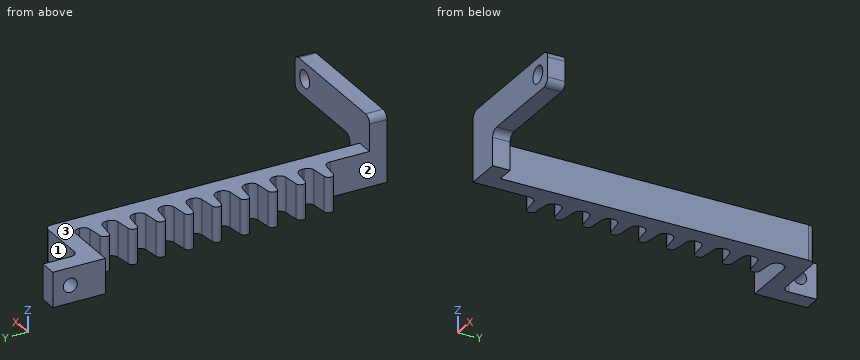
from build123d import *

# Parameters (mm, degrees)
BOSS_EXTRUDE1_DEPTH    = 7
SKETCH2_W              = 5
SKETCH2_H              = 10
BOSS_EXTRUDE2_DEPTH    = 95
SKETCH15_R             = 3.5
CUT_EXTRUDE3_DEPTH     = 7
SKETCH18_W             = 10
SKETCH18_H             = 5
BOSS_EXTRUDE3_DEPTH    = 34
BOSS_EXTRUDE4_DEPTH    = 10
FILLET1_R              = 2
FILLET2_R              = 2
LPATTERN2_COUNT        = 9
LPATTERN2_PITCH        = 8
FILLET1_OF_LPATTERN2_R = 2
SKETCH20_R             = 2.5
CUT_EXTRUDE4_DEPTH     = 10
CIRPATTERN2_COUNT      = 4
SKETCH22_W             = 135.679550384
SKETCH22_H             = 112.96527187
CUT_EXTRUDE5_DEPTH     = 61.740758688
BOSS_EXTRUDE5_START    = 5
SKETCH23_R             = 2.5
BOSS_EXTRUDE5_DEPTH    = 5
CUT_EXTRUDE6_START     = -10
CUT_EXTRUDE6_DEPTH     = 10
SKETCH27_W             = 10
SKETCH27_H             = 5
BOSS_EXTRUDE6_DEPTH    = 5
SKETCH28_W             = 5
SKETCH28_H             = 10
BOSS_EXTRUDE7_DEPTH    = 10
SKETCH29_R             = 2
CUT_EXTRUDE7_DEPTH     = 5
FILLET3_R              = 2


with BuildPart() as part:
    # Sketch1 → Boss-Extrude1 (new body)
    with BuildSketch(Plane(origin=(0, 0, 0), x_dir=(1, 0, 0), z_dir=(0, 1, 0))):
        with BuildLine():
            Line((-8, 56.940758688), (-8, 59.740758688))
            ThreePointArc((-8, 59.740758688), (-7.414213562, 61.154972251), (-6, 61.740758688))
            Line((-6, 61.740758688), (6, 61.740758688))
            ThreePointArc((6, 61.740758688), (7.414213562, 61.154972251), (8, 59.740758688))
            Line((8, 59.740758688), (8, 56.940758688))
            ThreePointArc((8, 56.940758688), (22.004297361, 53.123073119), (34.606342345, 45.920050844))
            Line((34.606342345, 45.920050844), (36.586241332, 47.899949831))
            ThreePointArc((36.586241332, 47.899949831), (38.000454895, 48.485736269), (39.414668457, 47.899949831))
            Line((39.414668457, 47.899949831), (47.899949831, 39.414668457))
            ThreePointArc((47.899949831, 39.414668457), (48.485736269, 38.000454895), (47.899949831, 36.586241332))
            Line((47.899949831, 36.586241332), (45.920050844, 34.606342345))
            ThreePointArc((45.920050844, 34.606342345), (53.123073119, 22.004297361), (56.940758688, 8))
            Line((56.940758688, 8), (59.740758688, 8))
            ThreePointArc((59.740758688, 8), (61.154972251, 7.414213562), (61.740758688, 6))
            Line((61.740758688, 6), (61.740758688, -6))
            ThreePointArc((61.740758688, -6), (61.154972251, -7.414213562), (59.740758688, -8))
            Line((59.740758688, -8), (56.940758688, -8))
            ThreePointArc((56.940758688, -8), (53.123073119, -22.004297361), (45.920050844, -34.606342345))
            Line((45.920050844, -34.606342345), (47.899949831, -36.586241332))
            ThreePointArc((47.899949831, -36.586241332), (48.485736269, -38.000454895), (47.899949831, -39.414668457))
            Line((47.899949831, -39.414668457), (39.414668457, -47.899949831))
            ThreePointArc((39.414668457, -47.899949831), (38.000454895, -48.485736269), (36.586241332, -47.899949831))
            Line((36.586241332, -47.899949831), (34.606342345, -45.920050844))
            ThreePointArc((34.606342345, -45.920050844), (22.004297361, -53.123073119), (8, -56.940758688))
            Line((8, -56.940758688), (8, -59.740758688))
            ThreePointArc((8, -59.740758688), (7.414213562, -61.154972251), (6, -61.740758688))
            Line((6, -61.740758688), (-6, -61.740758688))
            ThreePointArc((-6, -61.740758688), (-7.414213562, -61.154972251), (-8, -59.740758688))
            Line((-8, -59.740758688), (-8, -56.940758688))
            ThreePointArc((-8, -56.940758688), (-22.004297361, -53.123073119), (-34.606342345, -45.920050844))
            Line((-34.606342345, -45.920050844), (-36.586241332, -47.899949831))
            ThreePointArc((-36.586241332, -47.899949831), (-38.000454895, -48.485736269), (-39.414668457, -47.899949831))
            Line((-39.414668457, -47.899949831), (-47.899949831, -39.414668457))
            ThreePointArc((-47.899949831, -39.414668457), (-48.485736269, -38.000454895), (-47.899949831, -36.586241332))
            Line((-47.899949831, -36.586241332), (-45.920050844, -34.606342345))
            ThreePointArc((-45.920050844, -34.606342345), (-53.123073119, -22.004297361), (-56.940758688, -8))
            Line((-56.940758688, -8), (-59.740758688, -8))
            ThreePointArc((-59.740758688, -8), (-61.154972251, -7.414213562), (-61.740758688, -6))
            Line((-61.740758688, -6), (-61.740758688, 6))
            ThreePointArc((-61.740758688, 6), (-61.154972251, 7.414213562), (-59.740758688, 8))
            Line((-59.740758688, 8), (-56.940758688, 8))
            ThreePointArc((-56.940758688, 8), (-53.123073119, 22.004297361), (-45.920050844, 34.606342345))
            Line((-45.920050844, 34.606342345), (-47.899949831, 36.586241332))
            ThreePointArc((-47.899949831, 36.586241332), (-48.485736269, 38.000454895), (-47.899949831, 39.414668457))
            Line((-47.899949831, 39.414668457), (-39.414668457, 47.899949831))
            ThreePointArc((-39.414668457, 47.899949831), (-38.000454895, 48.485736269), (-36.586241332, 47.899949831))
            Line((-36.586241332, 47.899949831), (-34.606342345, 45.920050844))
            ThreePointArc((-34.606342345, 45.920050844), (-22.004297361, 53.123073119), (-8, 56.940758688))
        make_face()
    extrude(amount=BOSS_EXTRUDE1_DEPTH)

    # Sketch2 → Boss-Extrude2 (add)
    with BuildSketch(Plane(origin=(0, 7, 0), x_dir=(1, 0, 0), z_dir=(0, 1, 0))):
        with Locations((19.5, 10)):
            Rectangle(SKETCH2_W, SKETCH2_H)
        with Locations((-19.5, 10)):
            Rectangle(SKETCH2_W, SKETCH2_H)
    extrude(amount=BOSS_EXTRUDE2_DEPTH)

    # Sketch15 → Cut-Extrude3 (cut)
    with BuildSketch(Plane.XZ):
        with Locations(Location((0, 0, 0), (0, 0, 270))):
            Circle(SKETCH15_R)
    extrude(amount=-CUT_EXTRUDE3_DEPTH, mode=Mode.SUBTRACT)

    # Sketch18 → Boss-Extrude3 (add)
    with BuildSketch(Plane(origin=(-17, 0, 0), x_dir=(0, 0, -1), z_dir=(1, 0, 0))):
        with Locations((10, 99.5)):
            Rectangle(SKETCH18_W, SKETCH18_H)
    extrude(amount=BOSS_EXTRUDE3_DEPTH)

    # Sketch19 → Boss-Extrude4 (add)
    with BuildSketch(Plane(origin=(0, 0, -15), x_dir=(-1, 0, 0), z_dir=(0, 0, -1))):
        with BuildLine():
            Line((-17, 93), (-11.04472309, 92.26878394))
            ThreePointArc((-11.04472309, 92.26878394), (-9.922197884, 91), (-11.04472309, 89.73121606))
            Line((-11.04472309, 89.73121606), (-17, 89))
            Line((-17, 89), (-17, 93))
        make_face()
    boss_extrude4 = extrude(amount=-BOSS_EXTRUDE4_DEPTH)

    # Fillet1
    fillet1_edges = [part.edges().sort_by_distance(p)[0] for p in [
        (17, 89, -10),
        (17, 93, -10),
    ]]
    fillet(fillet1_edges, radius=FILLET1_R)

    # Fillet2
    fillet2_edges = [part.edges().sort_by_distance(p)[0] for p in [
        (22, 102, -10),
        (-22, 102, -10),
        (-17, 97, -10),
        (17, 97, -10),
    ]]
    fillet(fillet2_edges, radius=FILLET2_R)

    # LPattern2: Boss-Extrude4 ×9
    with Locations(*[(0, -i * LPATTERN2_PITCH, 0) for i in range(1, LPATTERN2_COUNT)]):
        add(boss_extrude4)

    # Fillet1 of LPattern2
    fillet1_of_lpattern2_edges = [part.edges().sort_by_distance(p)[0] for p in [
        (17, 81, -10),
        (17, 85, -10),
        (17, 73, -10),
        (17, 77, -10),
        (17, 65, -10),
        (17, 69, -10),
        (17, 57, -10),
        (17, 61, -10),
        (17, 49, -10),
        (17, 53, -10),
        (17, 41, -10),
        (17, 45, -10),
        (17, 33, -10),
        (17, 37, -10),
        (17, 25, -10),
        (17, 29, -10),
    ]]
    fillet(fillet1_of_lpattern2_edges, radius=FILLET1_OF_LPATTERN2_R)

    # Sketch20 → Cut-Extrude4 (cut)
    with BuildSketch(Plane(origin=(0, 7, 0), x_dir=(1, 0, 0), z_dir=(0, 1, 0))):
        with Locations(Location((0, 50, 0), (0, 0, 270))):
            Circle(SKETCH20_R)
    cut_extrude4 = extrude(amount=-CUT_EXTRUDE4_DEPTH, mode=Mode.SUBTRACT)

    # CirPattern2: Cut-Extrude4 ×4 about axis
    cirpattern2_axis = Axis((0, 0, 0), (0, 1, 0))
    for i in range(1, CIRPATTERN2_COUNT):
        add(cut_extrude4.rotate(cirpattern2_axis, i * 360 / CIRPATTERN2_COUNT), mode=Mode.SUBTRACT)

    # Sketch22 → Cut-Extrude5 (cut)
    with BuildSketch(Plane(origin=(0, 0, 0), x_dir=(0, 0, -1), z_dir=(1, 0, 0))):
        with Locations((-0.132373771, 50.371775874)):
            Rectangle(SKETCH22_W, SKETCH22_H)
    extrude(amount=-CUT_EXTRUDE5_DEPTH, mode=Mode.SUBTRACT)

    # Sketch23 → Boss-Extrude5 (add)
    with BuildSketch(Plane(origin=(0, 7, 0), x_dir=(1, 0, 0), z_dir=(0, 1, 0)).offset(BOSS_EXTRUDE5_START)):
        with BuildLine():
            Line((55, 3), (55, -2.687123684))
            ThreePointArc((55, -2.687123684), (54.414213562, -4.101337246), (53, -4.687123684))
            Line((53, -4.687123684), (19, -4.687123684))
            ThreePointArc((19, -4.687123684), (17.585786438, -4.101337246), (17, -2.687123684))
            Line((17, -2.687123684), (17, 5))
            Line((17, 5), (53, 5))
            ThreePointArc((53, 5), (54.414213562, 4.414213562), (55, 3))
        make_face()
        with Locations(Location((50, 0, 0), (0, 0, 270))):
            Circle(SKETCH23_R, mode=Mode.SUBTRACT)
    extrude(amount=-BOSS_EXTRUDE5_DEPTH)

    # Sketch26 → Cut-Extrude6 (cut)
    with BuildSketch(Plane(origin=(0, 7, 0), x_dir=(1, 0, 0), z_dir=(0, 1, 0)).offset(CUT_EXTRUDE6_START)):
        with BuildLine():
            Line((6, 61.740758688), (0, 61.740758688))
            Line((0, 61.740758688), (0, 52.5))
            ThreePointArc((0, 52.5), (2.5, 50), (0, 47.5))
            Line((0, 47.5), (0, 3.5))
            ThreePointArc((0, 3.5), (3.5, 0), (0, -3.5))
            Line((0, -3.5), (0, -47.5))
            ThreePointArc((0, -47.5), (2.5, -50), (0, -52.5))
            Line((0, -52.5), (0, -61.740758688))
            Line((0, -61.740758688), (6, -61.740758688))
            ThreePointArc((6, -61.740758688), (7.414213562, -61.154972251), (8, -59.740758688))
            Line((8, -59.740758688), (8, -56.940758688))
            ThreePointArc((8, -56.940758688), (22.004297361, -53.123073119), (34.606342345, -45.920050844))
            Line((34.606342345, -45.920050844), (36.586241332, -47.899949831))
            ThreePointArc((36.586241332, -47.899949831), (38.000454895, -48.485736269), (39.414668457, -47.899949831))
            Line((39.414668457, -47.899949831), (47.899949831, -39.414668457))
            ThreePointArc((47.899949831, -39.414668457), (48.485736269, -38.000454895), (47.899949831, -36.586241332))
            Line((47.899949831, -36.586241332), (45.920050844, -34.606342345))
            ThreePointArc((45.920050844, -34.606342345), (53.123073119, -22.004297361), (56.940758688, -8))
            Line((56.940758688, -8), (59.740758688, -8))
            ThreePointArc((59.740758688, -8), (61.154972251, -7.414213562), (61.740758688, -6))
            Line((61.740758688, -6), (61.740758688, 6))
            ThreePointArc((61.740758688, 6), (61.154972251, 7.414213562), (59.740758688, 8))
            Line((59.740758688, 8), (56.940758688, 8))
            ThreePointArc((56.940758688, 8), (53.123073119, 22.004297361), (45.920050844, 34.606342345))
            Line((45.920050844, 34.606342345), (47.899949831, 36.586241332))
            ThreePointArc((47.899949831, 36.586241332), (48.485736269, 38.000454895), (47.899949831, 39.414668457))
            Line((47.899949831, 39.414668457), (39.414668457, 47.899949831))
            ThreePointArc((39.414668457, 47.899949831), (38.000454895, 48.485736269), (36.586241332, 47.899949831))
            Line((36.586241332, 47.899949831), (34.606342345, 45.920050844))
            ThreePointArc((34.606342345, 45.920050844), (22.004297361, 53.123073119), (8, 56.940758688))
            Line((8, 56.940758688), (8, 59.740758688))
            ThreePointArc((8, 59.740758688), (7.414213562, 61.154972251), (6, 61.740758688))
        make_face()
    extrude(amount=CUT_EXTRUDE6_DEPTH, mode=Mode.SUBTRACT)

    # Sketch27 → Boss-Extrude6 (add)
    with BuildSketch(Plane(origin=(22, 0, 0), x_dir=(0, 0, -1), z_dir=(1, 0, 0))):
        with Locations((10, 9.5)):
            Rectangle(SKETCH27_W, SKETCH27_H)
    extrude(amount=BOSS_EXTRUDE6_DEPTH)

    # Sketch28 → Boss-Extrude7 (add)
    with BuildSketch(Plane(origin=(0, 102, 0), x_dir=(1, 0, 0), z_dir=(0, 1, 0))):
        with Locations((2.5, 10)):
            Rectangle(SKETCH28_W, SKETCH28_H)
    extrude(amount=BOSS_EXTRUDE7_DEPTH)

    # Sketch29 → Cut-Extrude7 (cut)
    with BuildSketch(Plane(origin=(5, 0, 0), x_dir=(0, 0, -1), z_dir=(1, 0, 0))):
        with Locations((10, 107)):
            Circle(SKETCH29_R)
    extrude(amount=-CUT_EXTRUDE7_DEPTH, mode=Mode.SUBTRACT)

    # Fillet3
    fillet3_edges = [part.edges().sort_by_distance(p)[0] for p in [
        (27, 9.5, -5),
        (5, 102, -10),
    ]]
    fillet(fillet3_edges, radius=FILLET3_R)


solid = part.part
Geometry check sheet. Reference: the model listing, model coordinates, mm. Face numbers are marked on the shaded views. A direction names the side the tool comes from. Give positions to 0.01 mm unless a question says otherwise; leave off trailing zeros. Write each loop counter-clockwise with the first axis right and the second up, starting at its lowest first coordinate (ties: lowest second). Pieces come first, ordered by that corner, then holes. Notation, with made-up numbers: (75, -12.5) - (87, -12.5) arc R7 ccw to (87, -8.5) - close; hole circle Ø5 at (-4.5, 73). An arc over 180 degrees is marked (long way). Put each result on its own line as item: value.
1. Set-up check for the marked faces 1, 2 and 3: record each of +Z, -Z, +X, -X, +Y, -Y from which the full face is reachable in a straight line by a thin tool's end or side.
Ans:
face 1: +Z, -Z, +X, +Y
face 2: +Z, -Z, -X, -Y
face 3: +Z, +X, -X, +Y
2. Sectioned sample at B-B, the plane y = 107. Enter the section's corners in (x, z), plus the area to 3 significant figures.
Ans:
outline: (0, -15) - (5, -15) - (5, -12) - (0, -12) - close; (0, -8) - (5, -8) - (5, -5) - (0, -5) - close
area: 30.0 mm²
3. Thickness scan on line 1 (X direction, y = 8.55, z = 0); line 2 (Y direction, x = 3.3, z = -10); line 3 (Y direction, x = 50, z = -3.75). Record the ranges inside material, lowest first.
Ans:
line 1: x = 17 to 47.5, 52.5 to 55
line 2: y = 97 to 105, 109 to 112
line 3: y = 7 to 12
4. Sectioned sample at D-D, the plane x = 40. Enter the section's corners in (y, z), plus the area to 3 significant figures.
Ans:
outline: (7, -5) - (12, -5) - (12, 4.69) - (7, 4.69) - close
area: 48.4 mm²
5. Sectioned sample at C-C, the plane y = 17. Enter the section's corners in (x, z).
Ans:
outline: (17, -15) - (22, -15) - (22, -5) - (17, -5) - close
6. Sectioned sample at A-A, the plane x = 50. Enter the section's corners in (y, z), plus the area to 3 significant figures.
Ans:
outline: (7, -5) - (12, -5) - (12, -2.5) - (7, -2.5) - close; (7, 2.5) - (12, 2.5) - (12, 4.69) - (7, 4.69) - close
area: 23.4 mm²
7. Go/stop test with flat-tipped pins: pin 1 (10 mm diameter, centred on y = 46.5, z = -7.5, fed in from -X); pin 2 (6 mm diameter, centred on x = 8.5, y = 37.5, fed in from +Z); pin 3 (11 mm diameter, centred on y = 65, z = -9.5, fed in from +X); pin 4 (3.5 mm diameter, centred on y = 107, z = -10, fed in from -X). Record where each tip stops, or that it passes through.
Ans:
pin 1: stops at x = 9.92
pin 2: stops at z = -5
pin 3: stops at x = 22
pin 4: passes through
